Autodesk Inventor part; units mm, degrees
ref_plane "YZ Plane" through (0, 0, 0) normal (1, 0, 0) x (0, 1, 0)
ref_plane "XZ Plane" through (0, 0, 0) normal (0, 1, 0) x (-1, 0, 0)
ref_plane "XY Plane" through (0, 0, 0) normal (0, 0, 1) x (1, 0, 0)
sketch "Skizze1" plane through (0, 0, 0) normal (0, 1, 0) x (-1, 0, 0)
  circle A0 centre (0, 0) radius 7
  circle A1 centre (0, 0) radius 3.8
  dimension "d0" = 14
  dimension "d1" = 7.6
extrude "Extrusion1" add sketch "Skizze1" along normal blind 3 draft -8
ref_plane "Arbeitsebene1" through (0, -0.6, 0) normal (0, -1, 0) x (1, 0, 0)
sketch "Skizze3" plane through (0, 0, 0) normal (0, -1, 0) x (1, 0, 0)
  circle A0 centre (0, 0) radius 7
  circle A1 centre (0, 0) radius 6.05
  dimension "d7" = 12.1
extrude "Extrusion3" add sketch "Skizze3" along normal blind 8 draft -1
properties part number "ESP32_M12_CCTVAdapter"
Source: CAD feature listing. Evaluate the final solid. Frame: model axes, mm. A direction names the side the tool comes from. Coordinates: 2 decimals unless noted, no trailing zeros. Loops run counter-clockwise (first coordinate to the right, second up) from the corner with the lowest first, then second, coordinate; pieces in that order, holes last. Notation, with made-up numbers: (8, 35) - (32, 35) arc R25 cw to (32, 58) - close; hole circle Ø3 at (55, 7). An arc over 180 degrees is marked (long way). One line per question, with ' | ' between items.
1) Section A-A, the plane y = -2. Return loops of the section in (x, z).
Report:
outline: circle Ø13.93 at (0, 0); hole circle Ø12.17 at (0, 0)
2) Line query: line 1 along Y through (x, z) = (4.5, -2); line 2 along X through (y, z) = (-4.75, 5.5); line 3 along X through (y, z) = (-5.5, 4.75). Output: solid intervals per line, ascending.
Report:
line 1: y = 0 to 3 | line 2: x = -4.19 to -2.71, 2.71 to 4.19 | line 3: x = -5.01 to -3.9, 3.9 to 5.01
3) Pull-direction query (Z, two-part tool) for faces 3 (the face through (6.61, -3.94, -2.08)), 4 (the face through (-4, -8, 5)), 5 (the face through (0.85, 0.854, -3.827)); classes: released by +Z, released by -Z, zero draft, split by the parting line, or undercut.
Report:
face 3: split by the parting line | face 4: zero draft | face 5: undercut
4) First-contact query: P1, Ø1.5, axis at y = 1, z = 0, coming from the +X side; P2, Ø2, axis at x = -1.5, z = 3, coming from the +Y side; P3, Ø1, axis at x = -4.5, z = -3, coming from the -Y side; P4, Ø6, axis at x = -0.5, z = -0.5, coming from the -Y side. Flat tips, straight axial feed; report the tip coordinate or a pass-through.
Report:
P1: stops at x = 6.96 | P2: stops at y = 3 | P3: stops at y = 0 | P4: passes through
5) Set-up query: faces 1 (the face through (-3, 0, 3)), 2 (the face through (0.866, 2.479, -6.595)). Return all of +Z, -Z, +X, -X, +Y, -Y with unobstructed straight access to the full face (end or side cutting, diameter ignored); none if empty.
Report:
face 1: -Y | face 2: +Y
